Input: part model. Units: mm. Frame: model coordinates. Face numbers are marked on the shaded views. A direction names the side the tool comes from. Coordinates: 2 decimals unless noted, no trailing zeros. Order: outer loops, then holes, each group sorted by start corner. A loop starts at its lowest first (then second) coordinate and runs counter-clockwise, first axis right, second up. Notation, with made-up numbers: (-16, 25) -> (-3, 25) arc R26 cw to (-3, 44) -> close; hole circle Ø1 at (87.5, -5.75). An arc over 180 degrees is marked (long way). Use one line per item in the form item = value. Start each with the question number.
1) Ray query, line 1 along X through (y, z) = (11, -6); line 2 along X through (y, z) = (2, -38); line 3 along Z through (x, y) = (6, 11). Return the intervals inside material, ascending.
2) Section query C-C on y = 5.5. Output: boundary loops of the cut face in (x, z) (3 decimals).
3) Access query for the marked faces 4, 5, 6 and 7. Directions: +Z, -Z, +X, -X, +Y, -Y. A direction counts if a zero-diameter tool reaches every point of the face in a straight line with its end or side. Return the directions, or none.
4) Section query D-D on z = -61.5. Output: boundary loops of the cut face in (x, y).
5) Pin query (flat end, axial travel): pin 1 (1.5 mm diameter, centred on x = 14, y = 19, fed in from +Z); pin 2 (5 mm diameter, centred on x = 7, z = -39.5, fed in from +Y); pin 3 (15 mm diameter, centred on x = 44.45, z = -38.1, fed in from +Y); pin 4 (10 mm diameter, centred on y = 18.5, z = -42, fed in from +X). Return the tip coordinate at first contact, or that it passes through.
6) Section query A-A on z = -38.1. Output: boundary loops of the cut face in (x, y).
7) Draft query along Z for the marked faces 1, 2 and 3. Return one class per face: pulls with the +Z half, pulls with the -Z half, needs draft (parallel to the pull), parting line crosses it, or undercut.
8) Section query B-B on x = 46. Output: boundary loops of the cut face in (y, z), then the cut area to 3 significant figures.
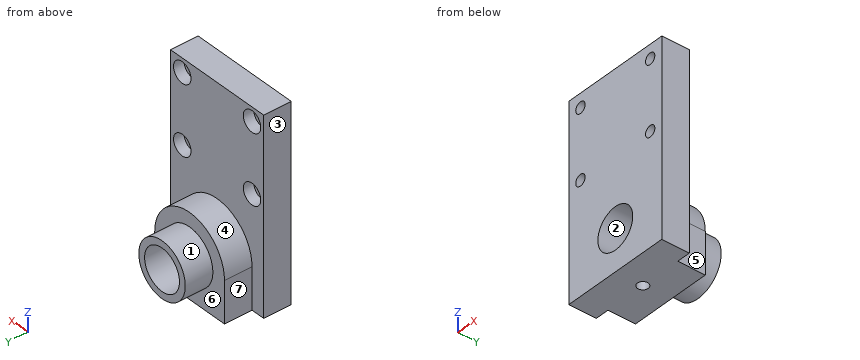
Autodesk Inventor part; units mm, degrees
ref_plane "YZ Plane" through (0, 0, 0) normal (1, 0, 0) x (0, 1, 0)
ref_plane "XZ Plane" through (0, 0, 0) normal (0, 1, 0) x (-1, 0, 0)
ref_plane "XY Plane" through (0, 0, 0) normal (0, 0, 1) x (1, 0, 0)
sketch "Sketch1" plane through (0, 0, 0) normal (0, 1, 0) x (-1, 0, 0)
  line L0 (0, 0) -> (-50.8, 0)
  line L1 (-50.8, 0) -> (-50.8, -88.9)
  line L2 (-50.8, -88.9) -> (0, -88.9)
  line L3 (0, -88.9) -> (0, 0)
  dimension "d0" = 50.8
  dimension "d1" = 88.9
extrude "Extrusion1" add sketch "Sketch1" along normal blind 12.7
sketch "Sketch2" plane through (0, 12.7, 0) normal (0, 1, 0) x (1, 0, 0)
  line L0 (50.8, 0) -> (50.8, 88.9)
  line L1 (50.8, 88.9) -> (0, 88.9)
  line L2 (0, 88.9) -> (0, 0)
  line L3 (6.35, 88.9) -> (44.45, 88.9)
  line L4 (44.45, 88.9) -> (44.45, 69.85)
  line L5 (44.45, 69.85) -> (6.35, 69.85)
  line L6 (6.35, 69.85) -> (6.35, 88.9)
  line L7 (6.35, 79.375) -> (0, 79.375) construction
  line L8 (44.45, 79.375) -> (50.8, 79.375) construction
  circle A0 centre (25.4, 69.85) radius 19.05
  dimension "d4" = 19.05
  dimension "d5" = 6.35
extrude "Extrusion2" add sketch "Sketch2" along normal blind 12.7
sketch "Sketch3" plane through (0, 25.4, 0) normal (0, 1, 0) x (1, 0, 0)
  arc A0 (6.35, 69.85) -> (44.45, 69.85) centre (25.4, 69.85) ccw
  circle A1 centre (25.4, 69.85) radius 12.7
  point P0 (0, 0)
  dimension "d8" = 25.4
extrude "Extrusion3" add sketch "Sketch3" along normal blind 12.7
sketch "Sketch6" plane through (0, 12.7, 0) normal (0, 1, 0) x (1, 0, 0)
  line L0 (0, 88.9) -> (0, 0)
  line L1 (0, 0) -> (50.8, 0)
  line L2 (50.8, 0) -> (50.8, 88.9)
  line L3 (44.45, 88.9) -> (44.45, 6.35) construction
  line L4 (44.45, 6.35) -> (6.35, 6.35) construction
  line L5 (6.35, 6.35) -> (6.35, 88.9) construction
  line L6 (6.35, 38.1) -> (44.45, 38.1) construction
  dimension "d35" = 6.35
  dimension "d36" = 31.75
hole "Hole3" at (25.4, 38.1, -69.85) direction (0, -1, 0) diameter 19.05 end through all
sketch "Sketch7" plane through (50.8, 0, -88.9) normal (0, 0, -1) x (-1, 0, 0)
  line L0 (0, 0) -> (0, 12.7)
  line L1 (44.45, 12.7) -> (6.35, 12.7) construction
  point P0 (25.4, 12.7)
hole "Hole4" at (25.4, 12.7, -88.9) direction (0, 0, 1) diameter 4.9784 end up to surface
hole "Hole5" at (6.35, 12.7, -6.35) at (6.35, 12.7, -38.1) at (44.45, 12.7, -6.35) at (44.45, 12.7, -38.1) direction (0, -1, 0) diameter 5.1054 end through all counterbore diameter 9.525 counterbore depth 4.826
properties part number "Holes Complete"
Answers below:
q1.line_1 = 0 to 1.6, 11.1 to 39.7, 49.2 to 50.8
q1.line_2 = 0 to 3.8, 8.9 to 41.9, 47 to 50.8
q1.line_3 = -88.9 to -42.85, -33.35 to -11.1, -1.6 to 0
q2.outline = (0, -88.9) -> (50.8, -88.9) -> (50.8, 0) -> (0, 0) -> close; hole circle Ø5.105 at (6.35, -38.1); hole circle Ø5.105 at (6.35, -6.35); hole circle Ø19.05 at (25.4, -69.85); hole circle Ø5.105 at (44.45, -38.1); hole circle Ø5.105 at (44.45, -6.35)
q3.face_4 = +Z, +Y
q3.face_5 = +Z, -Z, +X, +Y
q3.face_6 = +Y
q3.face_7 = +Z, -Z, -X, +Y
q4.outline = (0, 0) -> (20.82, 0) -> (20.82, 38.1) -> (15.83, 38.1) -> (15.83, 25.4) -> (8.28, 25.4) -> (8.28, 12.7) -> (0, 12.7) -> close; (29.98, 0) -> (50.8, 0) -> (50.8, 12.7) -> (42.52, 12.7) -> (42.52, 25.4) -> (34.97, 25.4) -> (34.97, 38.1) -> (29.98, 38.1) -> close
q5.pin_1 = -54.06
q5.pin_2 = 7.87
q5.pin_3 = 12.7
q5.pin_4 = through
q6.outline = (0, 0) -> (3.8, 0) -> (3.8, 7.87) -> (1.59, 7.87) -> (1.59, 12.7) -> (0, 12.7) -> close; (8.9, 0) -> (41.9, 0) -> (41.9, 7.87) -> (39.69, 7.87) -> (39.69, 12.7) -> (11.11, 12.7) -> (11.11, 7.87) -> (8.9, 7.87) -> close; (47, 0) -> (50.8, 0) -> (50.8, 12.7) -> (49.21, 12.7) -> (49.21, 7.87) -> (47, 7.87) -> close
q7.face_1 = parting line crosses it
q7.face_2 = undercut
q7.face_3 = needs draft
q8.outline = (0, -88.9) -> (12.7, -88.9) -> (12.7, -42.6) -> (7.87, -42.6) -> (7.87, -40.13) -> (0, -40.13) -> close; (0, -36.07) -> (7.87, -36.07) -> (7.87, -33.6) -> (12.7, -33.6) -> (12.7, -10.85) -> (7.87, -10.85) -> (7.87, -8.38) -> (0, -8.38) -> close; (0, -4.32) -> (7.87, -4.32) -> (7.87, -1.85) -> (12.7, -1.85) -> (12.7, 0) -> (0, 0) -> close
q8.area = 978 mm^2
